Geometry: final body of the model. Coordinates: model frame, mm. Coordinates: 2 decimals unless noted, no trailing zeros. Loops run counter-clockwise (first coordinate to the right, second up) from the corner with the lowest first, then second, coordinate; pieces in that order, holes last. Notation, with made-up numbers: (-31.5, 22) - (-19.5, 22) arc R21 ccw to (-19.5, 33) - close; hole circle Ø5 at (43.25, -6.75). An arc over 180 degrees is marked (long way). Put each result on its own line as item: value. Start each with the question number.
1) Section A-A on x = 0. Output: boundary loops of the cut face in (y, z) (1 decimal).
2) Material intervals for line 1 along Y through (x, z) = (-1, 3.25) (3 decimals); line 2 along Z through (x, y) = (0.5, -50.5); line 3 along X through (y, z) = (-78, 1), sorted ascending. Write a range as from..to.
3) Section C-C on z = -4. Output: boundary loops of the cut face in (x, y) (3 decimals).
4) Contact query for flat-ended pins moving along their axis: pin 1 Ø0.9 at (x, y) = (0.5, -55) entering from +Z; pin 2 Ø10 at (y, z) = (-84, 7) entering from -X; pin 3 Ø0.9 at (x, y) = (0, -53) entering from +Z; pin 4 Ø12 at (y, z) = (-37.5, -6) entering from -X. Output: stop coordinate, or through.
5) Section D-D on y = -34.5. Output: boundary loops of the cut face in (x, z).
6) Section B-B on y = -48.5. Output: boundary loops of the cut face in (x, z).
```python
from build123d import *

# Parameters (mm, degrees)
F0_R      = 1.5
F1_DEPTH  = 101.6
F2_R      = 10.4851931458
F3_DEPTH  = 3.175
F4_W      = 10.1616978645
F4_H      = 12.8714852035
F5_DEPTH  = 20.24025
F7_DEPTH  = 8.96719
F9_W      = 3
F9_H      = 3.249252215
F10_DEPTH = 0.77209


with BuildPart() as f1:
    # F0 (on Front) → F1 (new body)
    with BuildSketch(Plane.XZ):
        Circle(F0_R)
    extrude(amount=F1_DEPTH)

    # F2 (on face) → F3 (join)
    with BuildSketch(Plane.XZ.offset(101.6)):
        Circle(F2_R)
    extrude(amount=F3_DEPTH)

    # F4 (on Top) → F5 (cut)
    with BuildSketch(Plane.XY):
        with Locations((0, -50.7002491504)):
            Rectangle(F4_W, F4_H)
    extrude(amount=F5_DEPTH, mode=Mode.SUBTRACT)

    # F9 (on face) → F10 (join)
    with BuildSketch(Plane.XY):
        with Locations((0, -52.3248752579)):
            Rectangle(F9_W, F9_H)
    extrude(amount=F10_DEPTH)


with BuildPart() as f7:
    # F6 (on face) → F7 (new body)
    with BuildSketch(Plane.XZ.offset(44.2645065486)):
        with BuildLine():
            Line((0.595669005, 1.3766547993), (-0.595669005, 1.3766547993))
            Line((-0.595669005, 1.3766547993), (-0.595669005, 0.1358163867))
            Line((-0.595669005, 0.1358163867), (1.3222411928, 0.1358163867))
            Line((1.3222411928, 0.1358163867), (1.3222411928, 0.7082924736))
            ThreePointArc((1.3222411928, 0.7082924736), (1.0155155987, 1.1039601753), (0.595669005, 1.3766547993))
        make_face()
        with BuildLine():
            Line((1.3222411928, 1.3766547993), (0.595669005, 1.3766547993))
            ThreePointArc((0.595669005, 1.3766547993), (1.0155155987, 1.1039601753), (1.3222411928, 0.7082924736))
            Line((1.3222411928, 0.7082924736), (1.3222411928, 1.3766547993))
        make_face()
    extrude(amount=F7_DEPTH)


solid = f1.part
```
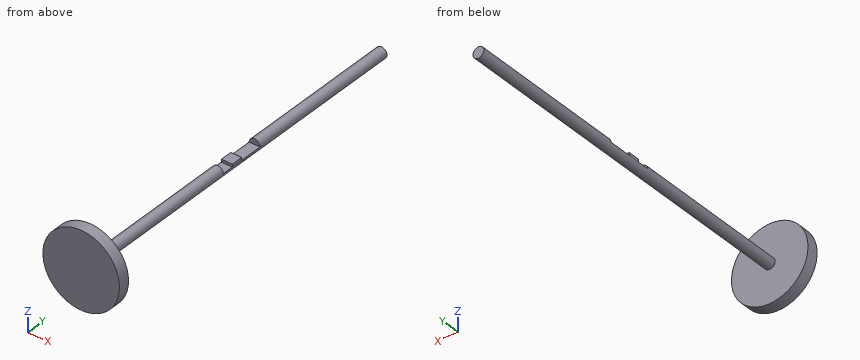
Answer block:
1. outline: (-104.8, -10.5) - (-101.6, -10.5) - (-101.6, -1.5) - (0, -1.5) - (0, 1.5) - (-44.3, 1.5) - (-44.3, 0) - (-50.7, 0) - (-50.7, 0.8) - (-53.9, 0.8) - (-53.9, 0) - (-57.1, 0) - (-57.1, 1.5) - (-101.6, 1.5) - (-101.6, 10.5) - (-104.8, 10.5) - close
2. line 1: y = -104.775..-101.6
2. line 2: z = -1.41..0
2. line 3: x = -1.12..1.12
3. outline: (-9.692, -104.775) - (9.692, -104.775) - (9.692, -101.6) - (-9.692, -101.6) - close
4. pin 1: stops at z = 0
4. pin 2: passes through
4. pin 3: stops at z = 0.77
4. pin 4: stops at x = -1.5
5. outline: circle Ø3 at (0, 0)
6. outline: (-1.5, 0) arc R1.5 ccw to (1.5, 0) - close
